from build123d import *

# Parameters (mm, degrees)
BOSS_EXTRUDE1_DEPTH = 5
BOSS_EXTRUDE2_START = -5
BOSS_EXTRUDE2_DEPTH = 2
FILLET1_R           = 5
FILLET2_R           = 1
FILLET3_R           = 1
CUT_EXTRUDE1_DEPTH  = 63.739091162
FILLET4_R           = 0.5


with BuildPart() as part:
    # Sketch32 → Boss-Extrude1 (new body)
    with BuildSketch(Plane(origin=(0, 0, 0), x_dir=(0, 0, -1), z_dir=(1, 0, 0))):
        Polygon((-23.663373299, 32.245792092), (-0.6, 4.759934105), (-0.6, 58.641752364), align=None)
    extrude(amount=-BOSS_EXTRUDE1_DEPTH)

    # Sketch33 → Boss-Extrude2 (add)
    with BuildSketch(Plane(origin=(0, 0, 0), x_dir=(0, 0, -1), z_dir=(1, 0, 0)).offset(BOSS_EXTRUDE2_START)):
        Polygon((0, 0), (2, 0), (2, 63.28), (0, 63.28), (-27.086136094, 32.28), align=None)
    extrude(amount=BOSS_EXTRUDE2_DEPTH)

    # Fillet1
    fillet1_edges = [part.edges().sort_by_distance(p)[0] for p in [
        (-4, 32.28, 27.086136094),
    ]]
    fillet(fillet1_edges, radius=FILLET1_R)

    # Fillet2
    fillet2_edges = [part.edges().sort_by_distance(p)[0] for p in [
        (-1.5, 4.759934105, 0.6),
        (-1.5, 58.641752364, 0.6),
        (-1.5, 32.245792092, 23.663373299),
    ]]
    fillet(fillet2_edges, radius=FILLET2_R)

    # Fillet3
    fillet3_edges = [part.edges().sort_by_distance(p)[0] for p in [
        (-4, 63.28, -2),
        (-4, 63.28, 0),
        (-4, 0, 0),
        (-4, 0, -2),
    ]]
    fillet(fillet3_edges, radius=FILLET3_R)


with BuildPart() as part_1:
    # Body-Move/Copy1: moved
    add(part.part.moved(Location((20.819939299, -2.965088501, -8.971960843))))

    # Sketch34 → Cut-Extrude1 (cut, through all)
    with BuildSketch(Plane.ZY.offset(-15.819939299)):
        with BuildLine():
            Line((14.128009591, 29.925516449), (11.361881222, 33.091341915))
            Line((11.361881222, 33.091341915), (-8.371960843, 9.573464739))
            Line((-8.371960843, 9.573464739), (-8.371960843, 4.542323024))
            ThreePointArc((-8.371960843, 4.542323024), (-7.713980986, 3.602630403), (-6.6059164, 3.899535414))
            Line((-6.6059164, 3.899535414), (13.428952617, 27.776162543))
            Line((13.428952617, 27.776162543), (14.14100967, 28.624759093))
            ThreePointArc((14.14100967, 28.624759093), (14.374915288, 29.277540443), (14.128009591, 29.925516449))
        make_face()
    extrude(amount=-CUT_EXTRUDE1_DEPTH, mode=Mode.SUBTRACT)

    # Fillet4
    fillet4_edges = [part_1.edges().sort_by_distance(p)[0] for p in [
        (19.319939299, 33.091341915, 11.361881222),
        (19.319939299, 9.573464739, -8.371960843),
    ]]
    fillet(fillet4_edges, radius=FILLET4_R)


solid = part_1.part
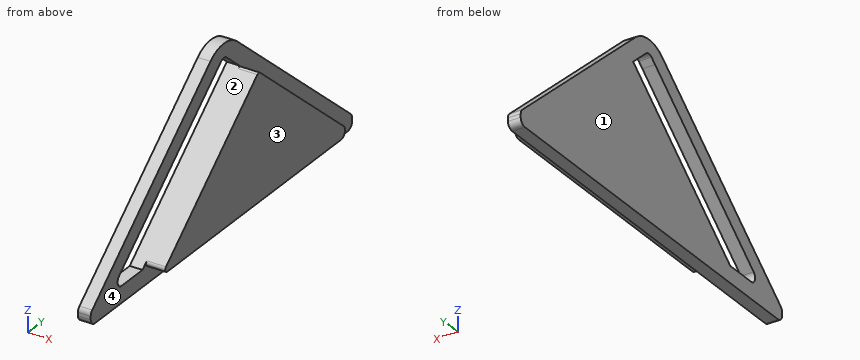
Geometry check sheet. Reference: the model listing, model coordinates, mm. Face numbers are marked on the shaded views. A direction names the side the tool comes from. Give positions to 0.01 mm unless a question says otherwise; leave off trailing zeros. Order: outer loops, then holes, each group sorted by start corner. A loop starts at its lowest first (then second) coordinate and runs counter-clockwise, first axis right, second up. Notation, with made-up numbers: (71.5, 0) - (106.5, 0) arc R23 ccw to (106.5, 34) - close; hole circle Ø10 at (-30, 68.25). An arc over 180 degrees is marked (long way). Answer as a JSON object with one key per item and string values.
(1) Material ranges on line 1 (X direction, y = 30.5, z = 14.75); line 2 (Y direction, x = 17.75, z = 0.75); line 3 (Y direction, x = 16.1, z = 8.25), recorded low to high.
Report:
{"line 1": "15.82 to 17.82", "line 2": "8.62 to 12.67, 20.44 to 49.19", "line 3": "17.56 to 21.6, 29.38 to 40.6"}
(2) Cross-section at B-B (x = 16.5). Record the cut outline in (y, z), then the cut area to 3 significant figures.
Report:
{"outline": "(-2.97, -9.97) arc R1 ccw to (-1.97, -10.97) - (59.31, -10.97) arc R1 ccw to (60.31, -9.97) - (60.31, -9.43) arc R1 ccw to (59.97, -8.67) - (32.54, 15.3) arc R5 ccw to (26.04, 15.36) - (-2.61, -8.67) arc R1 ccw to (-2.97, -9.44) - close; hole (3.9, -6.61) arc R1 ccw to (4.54, -8.37) - (9.57, -8.37) - (33.09, 11.36) - (29.93, 14.13) arc R1 ccw to (28.62, 14.14) - close", "area": "815 mm^2"}
(3) Draft check along Z on the marked faces 1 and 2. Enter one of: released by +Z, released by -Z, zero draft, split by the parting line, or undercut.
Report:
{"face 1": "zero draft", "face 2": "undercut"}
(4) Depth check by flat-ended pin: pin 1 Ø4 at (y, z) = (12.5, 8.5) entering from -X; pin 2 Ø8 at (y, z) = (52, -4.5) entering from +X; pin 3 Ø2 at (x, y) = (16.5, 8) entering from +Z; pin 4 Ø1.5 at (x, y) = (20, 34.5) entering from -Z. Enter the tip coordinate at first touch or a pass-through.
Report:
{"pin 1": "through", "pin 2": "x = 20.82", "pin 3": "z = 1.07", "pin 4": "z = -8.37"}
(5) Tool access check on the marked faces 3 and 4. Record the directions out of +Z, -Z, +X, -X, +Y, -Y that give a thin tool (end or side, any length) a straight path to the whole face; none if there is none.
Report:
{"face 3": "+Z, -Z, +X, +Y, -Y", "face 4": "+X"}
(6) Cross-section at C-C (y = 6). Record the cut outline in (x, z).
Report:
{"outline": "(15.82, -10.97) - (17.82, -10.97) - (17.82, -8.37) - (15.82, -8.37) - close; (15.82, -4.84) - (17.82, -4.84) - (17.82, -1.45) - (15.82, -1.45) - close"}
(7) Cross-section at A-A (z = -5.5). Record the cut outline in (x, y), then the cut area to 3 significant figures.
Report:
{"outline": "(15.82, 1.17) - (17.82, 1.17) - (17.82, 5.22) - (15.82, 5.22) - close; (15.82, 13) - (20.82, 13) - (20.82, 52.39) - (17.82, 52.39) - (17.82, 56.34) - (15.82, 56.34) - close", "area": "213 mm^2"}
(8) Cross-section at D-D (y = 36). Record the cut outline in (x, z), then the cut area to 3 significant figures.
Report:
{"outline": "(15.82, -10.97) - (17.82, -10.97) - (17.82, -8.37) - (20.82, -8.37) - (20.82, 8.82) - (17.82, 8.82) - (17.82, 12.27) - (15.82, 12.27) - close", "area": "98.1 mm^2"}
